Autodesk Inventor part; units mm, degrees
ref_plane "Work Plane1" through (0.508, 0.508, 2.286) normal (0, 0, 1) x (1, 0, 0)
ref_plane "Work Plane2" through (0.508, 0.508, 2.286) normal (0, 0, 1) x (1, 0, 0)
ref_plane "Work Plane3" through (0.508, 0.508, 4.826) normal (0, 0, 1) x (1, 0, 0)
sketch "Sketch1" plane through (0, 0, 0) normal (0, 0, 1) x (1, 0, 0)
  line L0 (0, 87.3125) -> (163.83, 87.3125)
  line L1 (163.83, 87.3125) -> (163.83, 0)
  line L2 (163.83, 0) -> (0, 0)
  line L3 (0, 0) -> (0, 87.3125)
  dimension "d0" = 163.83
  dimension "d1" = 87.3125
extrude "Extrusion1" add sketch "Sketch1" along normal blind 2.54
sketch "Sketch2" plane through (0, 0, 2.54) normal (0, 0, 1) x (1, 0, 0)
  point P0 (0, 0)
fillet "Fillet1" radius 20.6375 1 edges at (163.83, 87.3125, 1.27)
fillet "Fillet2" radius 20.6375 1 edges at (0, 87.3125, 1.27)
sketch "Sketch8" plane through (0, 0, 2.54) normal (0, 0, 1) x (1, 0, 0)
  point P0 (0, 0)
sketch "Sketch11" plane through (0, 0, 2.54) normal (0, 0, 1) x (1, 0, 0)
  point P0 (0, 0)
sketch "Sketch15" plane through (0, 0, 2.54) normal (0, 0, 1) x (1, 0, 0)
  line L0 (83.566, 56.2102) -> (136.1122, 56.2102)
  line L1 (136.1122, 56.2102) -> (136.1122, 16.51)
  line L2 (136.1122, 16.51) -> (83.566, 16.51)
  line L3 (83.566, 16.51) -> (83.566, 56.2102)
  line L4 (0, 0) -> (163.83, 0)
  line L5 (163.83, 0) -> (163.83, 66.675)
  dimension "d136" = 52.5463
  dimension "d137" = 16.51
  dimension "d151" = 39.7002
  dimension "d184" = 27.7177
extrude "Extrusion6" add sketch "Sketch15" along normal blind 5.08
shell "Shell5" thickness 0.762 removed faces 1 at (101.0814, 42.9768, 7.62)
sketch "Sketch16" plane through (0, 0, 2.54) normal (0, 0, 1) x (1, 0, 0)
  line L0 (103.124, 82.5754) -> (135.89, 82.5754)
  line L1 (135.89, 82.5754) -> (135.89, 56.2102)
  line L2 (135.89, 56.2102) -> (103.124, 56.2102)
  line L3 (103.124, 56.2102) -> (103.124, 82.5754)
  arc A0 (163.83, 66.675) -> (143.1925, 87.3125) centre (143.1925, 66.675) ccw
  line L4 (136.1122, 56.2102) -> (83.566, 56.2102)
  point P0 (0, 0)
  dimension "d62" = 32.766
  dimension "d63" = 26.3652
  dimension "d183" = 27.94
  dimension "d231" = 0
extrude "Extrusion7" add sketch "Sketch16" along normal blind 5.08
shell "Shell6" thickness 0.762 removed faces 1 at (124.968, 73.787, 7.62)
sketch "Sketch20" plane through (0, 0, 2.54) normal (0, 0, 1) x (1, 0, 0)
  circle A0 centre (60.325, 76.2) radius 4.445
  line L0 (0, 66.675) -> (0, 0)
  line L1 (103.124, 87.3125) -> (20.6375, 87.3125)
  point P0 (103.124, 82.5754)
  point P1 (20.6375, 87.3125)
  dimension "d77" = 8.89
  dimension "d138" = 60.325
  dimension "d150" = 11.1125
sketch "Sketch24" plane through (0, 0, 2.54) normal (0, 0, 1) x (1, 0, 0)
  line L0 (0, 0) -> (83.7565, 0)
  line L1 (83.7565, 0) -> (83.7565, 66.3575)
  line L2 (83.7565, 66.3575) -> (0, 66.3575)
  line L3 (0, 66.3575) -> (0, 0)
  line L4 (103.124, 87.3125) -> (20.6375, 87.3125)
  point P0 (103.124, 82.5754)
  point P1 (20.6375, 87.3125)
  dimension "d114" = 83.7565
  dimension "d210" = 20.955
extrude "Extrusion13" add sketch "Sketch24" along normal blind 7.62
sketch "Sketch25" plane through (0, 0, 2.54) normal (0, 0, 1) x (1, 0, 0)
  circle A0 centre (57.2977, 68.2625) radius 1.5875
  line L0 (0, 66.675) -> (0, 66.3575)
  circle A1 centre (63.6477, 68.2625) radius 1.5875
  line L1 (103.124, 87.3125) -> (20.6375, 87.3125)
  point P0 (0, 0)
  point P1 (103.124, 82.5754)
  point P2 (20.6375, 87.3125)
  dimension "d126" = 3.175
  dimension "d139" = 57.2977
  dimension "d141" = 6.35
  dimension "d149" = 19.05
sketch "Sketch27" plane through (0, 0, 2.54) normal (0, 0, 1) x (1, 0, 0)
  line L0 (62.5475, 79.375) -> (72.7075, 79.375)
  line L1 (72.7075, 79.375) -> (72.7075, 73.025)
  line L2 (72.7075, 73.025) -> (62.5475, 73.025)
  line L3 (62.5475, 73.025) -> (62.5475, 79.375)
  arc A0 (20.6375, 87.3125) -> (0, 66.675) centre (20.6375, 66.675) ccw
  point P0 (0, 0)
  dimension "d181" = 41.91
  dimension "d182" = 10.16
ref_plane "Work Plane1" through (0.508, 0.508, 2.286) normal (0, 0, 1) x (1, 0, 0)
sketch "Sketch28" plane through (0.508, 0.508, 2.286) normal (0, 0, 1) x (1, 0, 0)
  circle A0 centre (57.15, 48.7045) radius 1.5875
  circle A1 centre (56.7897, 67.7545) radius 1.5875
  circle A2 centre (63.5, 48.7045) radius 1.5875
  circle A3 centre (62.992, 67.7545) radius 1.5875
  point P0 (-0.508, -0.508)
  dimension "d154" = 19.05
  dimension "d155" = 3.175
  dimension "d156" = 19.05
  dimension "d157" = 6.35
ref_plane "Work Plane2" through (0.508, 0.508, 2.286) normal (0, 0, 1) x (1, 0, 0)
sketch "Sketch29" plane through (0.508, 0.508, 2.286) normal (0, 0, 1) x (1, 0, 0)
  line L0 (82.7405, 64.7065) -> (0, 64.7065)
  line L1 (82.7405, 0) -> (0, 0)
  line L2 (0, 64.7065) -> (82.7405, 64.7065)
  line L3 (82.7405, 64.7065) -> (82.7405, 0)
  line L4 (82.7405, 0) -> (0, 0)
  line L5 (0, 0) -> (0, 64.7065)
  point P0 (-0.508, -0.508)
  point P1 (84.836, 62.484)
extrude "Extrusion16" add sketch "Sketch29" along normal blind 2.54
ref_plane "Work Plane3" through (0.508, 0.508, 4.826) normal (0, 0, 1) x (1, 0, 0)
sketch "Sketch30" plane through (0.508, 0.508, 4.826) normal (0, 0, 1) x (1, 0, 0)
  circle A0 centre (57.15, 48.7045) radius 3.175
  circle A1 centre (63.5, 48.7045) radius 3.175
  circle A2 centre (56.7897, 67.7545) radius 1.5875
  circle A3 centre (62.992, 67.7545) radius 1.5875
  point P0 (-0.508, -0.508)
  dimension "d162" = 6.35
  dimension "d163" = 19.05
  dimension "d164" = 19.05
sketch "Sketch33" plane through (20.6375, 86.5505, 0.762) normal (0, 0, 1) x (1, 0, 0)
  line L0 (63.6905, -69.2785) -> (63.6905, -31.1023)
  line L1 (114.7127, -69.2785) -> (63.6905, -69.2785)
  line L2 (63.6905, -31.1023) -> (114.7127, -31.1023)
  line L3 (114.7127, -31.1023) -> (114.7127, -69.2785)
  line L4 (114.7127, -69.2785) -> (63.6905, -69.2785)
  line L5 (63.6905, -69.2785) -> (63.6905, -31.1023)
  point P0 (-20.6375, -86.5505)
extrude "Extrusion20" add sketch "Sketch33" along normal blind 1.778
sketch "Sketch34" plane through (0, 0, 0) normal (0, 0, -1) x (-1, 0, 0)
  line L0 (-163.83, 0) -> (0, 0)
  line L1 (0, 0) -> (0, 87.3125)
  line L2 (0, 87.3125) -> (-163.83, 87.3125)
  line L3 (-163.83, 87.3125) -> (-163.83, 0)
  point P0 (0, 0)
extrude "Extrusion21" add sketch "Sketch34" against normal blind 2.54
extrude "Extrusion22" cut sketch "Sketch20" against normal blind 7.62
extrude "Extrusion23" cut sketch "Sketch25" against normal blind 7.62
extrude "Extrusion24" cut sketch "Sketch28" along normal mid plane 7.62 contours A0 | A2
extrude "Extrusion25" cut sketch "Sketch27" against normal blind 7.62
fillet "Fillet4" radius 20.6375 1 edges at (163.83, 87.3125, 1.27)
fillet "Fillet5" radius 20.6375 1 edges at (0, 87.3125, 1.27)
sketch "Sketch35" plane through (0, 0, 2.54) normal (0, 0, 1) x (1, 0, 0)
  line L0 (135.3502, 17.272) -> (84.328, 17.272)
  line L1 (135.3502, 17.272) -> (162.2742, 17.272)
  line L2 (162.2742, 17.272) -> (162.2742, 66.802)
  line L3 (162.2742, 66.802) -> (135.3502, 66.802)
  line L4 (135.3502, 66.802) -> (135.3502, 17.272)
  point P0 (0, 0)
  point P1 (85.344, 22.352)
  dimension "d199" = 26.924
  dimension "d200" = 49.53
extrude "Extrusion26" add sketch "Sketch35" along normal blind 5.08
sketch "Sketch36" plane through (0, 0, 7.62) normal (0, 0, 1) x (1, 0, 0)
  line L0 (136.6202, 65.532) -> (160.4327, 65.532)
  line L1 (160.4327, 65.532) -> (160.4327, 14.732)
  line L2 (160.4327, 14.732) -> (136.6202, 14.732)
  line L3 (136.6202, 14.732) -> (136.6202, 65.532)
  line L4 (135.3502, 55.4482) -> (135.3502, 17.272)
  line L5 (162.2742, 66.802) -> (135.89, 66.802)
  line L6 (136.1122, 17.272) -> (162.2742, 17.272)
  point P0 (0, 0)
  point P1 (135.3502, 66.802)
  dimension "d203" = 23.8125
  dimension "d204" = 1.27
  dimension "d205" = 1.27
  dimension "d207" = 50.8
extrude "Extrusion27" cut sketch "Sketch36" against normal blind 5.08
sketch "Sketch37" plane through (0, 0, 10.16) normal (0, 0, 1) x (1, 0, 0)
  line L0 (0.762, 3.048) -> (83.5152, 3.048)
  line L1 (83.5152, 3.048) -> (83.5152, 65.3859)
  line L2 (83.5152, 65.3859) -> (0.762, 65.386)
  line L3 (0.762, 65.386) -> (0.762, 3.048)
  line L4 (0, 66.3575) -> (0, 0)
  line L5 (0, 0) -> (83.7565, 0)
  dimension "d211" = 82.7532
  dimension "d212" = 62.3379
  dimension "d213" = 0.762
  dimension "d214" = 3.048
extrude "Extrusion28" cut sketch "Sketch37" against normal blind 7.62
extrude "Extrusion29" cut sketch "Sketch30" against normal blind 2.54 contours A0 | A1
sketch "Sketch38" plane through (0, 0, 2.54) normal (0, 0, 1) x (1, 0, 0)
  line L0 (163.83, 0) -> (0, 0)
  line L1 (163.83, 0) -> (84.1375, 0)
  line L2 (84.1375, 0) -> (84.1375, 16.51)
  line L3 (84.1375, 16.51) -> (163.83, 16.51)
  line L4 (163.83, 16.51) -> (163.83, 0)
  dimension "d229" = 16.51
extrude "Extrusion30" cut sketch "Sketch38" against normal blind 12.7
sketch "Sketch39" plane through (0, 0, 7.62) normal (0, 0, 1) x (1, 0, 0)
  line L0 (83.7565, 66.3575) -> (83.7565, 56.2102)
  line L1 (83.7565, 56.2102) -> (84.328, 56.2102)
  line L2 (84.328, 56.2102) -> (84.328, 0)
  line L3 (84.328, 0) -> (83.7565, 0)
  line L4 (83.7565, 0) -> (83.7565, 56.2102)
  line L5 (84.328, 17.272) -> (84.328, 55.4482)
  line L6 (83.7565, 0) -> (84.1375, 0)
  point P0 (0, 0)
  dimension "d221" = 0
  dimension "d230" = 0
extrude "Extrusion31" add sketch "Sketch39" along normal blind 2.54 and the other way blind 7.62
sketch "Sketch40" plane through (0, 0, 10.16) normal (0, 0, 1) x (1, 0, 0)
  line L0 (84.328, 0) -> (84.328, 56.2102)
  line L1 (0, 0) -> (84.328, 0)
  line L2 (84.328, 0) -> (84.328, 2.032)
  line L3 (84.328, 2.032) -> (0, 2.032)
  line L4 (0, 2.032) -> (0, 0)
  line L5 (83.5152, 3.048) -> (0.762, 3.048)
  dimension "d226" = 1.016
extrude "Extrusion32" cut sketch "Sketch40" against normal blind 12.7
properties part number "Base Plate 2"
Geometry check sheet. Reference: the model listing, model coordinates, mm. A direction names the side the tool comes from. Round coordinates to 2 decimals unless told otherwise and drop trailing zeros. Loops run counter-clockwise (first coordinate to the right, second up) from the corner with the lowest first, then second, coordinate; pieces in that order, holes last. Notation, with made-up numbers: (70, 29.5) - (121, 29.5) arc R12 cw to (121, 36.5) - close; hole circle Ø3 at (33, 7.5). An arc over 180 degrees is marked (long way). Write item = value, one per line. Start each with the question number.
1. Section check D-D on x = 78. Enter the section's corners in (y, z), then the cut area to 3 significant figures.
2. Thickness scan on line 1 (Y direction, x = 109.5, z = 4.5); line 2 (X direction, y = 52.5, z = 7.5); line 3 (X direction, y = 65.5, z = 3.5). Record the ranges inside material, lowest first.
3. Section check A-A on z = 5.25. Give the number of separate pieces and of enclosed holes in the cut face, then the cut area to 3 significant figures.
4. Depth check by flat-ended pin: pin 1 (6 mm diameter, centred on y = 22.5, z = 8, fed in from -X); pin 2 (6 mm diameter, centred on x = 52.5, z = 7, fed in from +Y); pin 3 (2.5 mm diameter, centred on y = 52.5, z = 5, fed in from +X); pin 4 (2.5 mm diameter, centred on x = 63.65, y = 68.26, fed in from +Z). Enter the tip coordinate at first touch or a pass-through.
5. Section check B-B on y = 76.2. Enter the section's corners in (x, z), then the cut area to 3 significant figures.
6. Set-up check for faces 1 (the face through (119, 82.575, 5)), 2 (the face through (110, 17.272, 5)), 3 (the face through (161, 42, 7.62)), 4 (the face through (83.756, 61, 6)): record each of +Z, -Z, +X, -X, +Y, -Y from which the full face is reachable in a straight line by a thin tool's end or side.
7. Mould release check, pull along Y, two halves, no side actions. Record for faces 5 (the face through (136.62, 41, 5)), 6 (the face through (148, 65.532, 5)), 7 (the face through (42, 35, 2.54)): released by +Y, released by -Y, zero draft, split by the parting line, or undercut.
8. Section check C-C on y = 22.5. Enter the section's corners in (x, z).
Working result:
q1.outline = (2.03, 0) - (87.31, 0) - (87.31, 2.54) - (66.36, 2.54) - (66.36, 10.16) - (65.39, 10.16) - (65.39, 2.54) - (3.05, 2.54) - (3.05, 10.16) - (2.03, 10.16) - close
q1.area = 232 mm^2
q2.line_1 = 16.51 to 17.27, 55.45 to 56.21, 81.81 to 82.58
q2.line_2 = 0 to 0.76, 83.52 to 84.33, 135.35 to 136.62, 160.43 to 162.27
q2.line_3 = 0 to 83.76, 103.12 to 103.89, 135.13 to 136.62, 160.43 to 162.27
q3.separate_pieces = 1
q3.enclosed_holes = 3
q3.area = 581 mm^2
q4.pin_1 = 0
q4.pin_2 = 66.36
q4.pin_3 = 162.27
q4.pin_4 = through
q5.outline = (2.33, 0) - (55.88, 0) - (55.88, 2.54) - (2.33, 2.54) - close; (72.71, 0) - (161.5, 0) - (161.5, 2.54) - (135.89, 2.54) - (135.89, 7.62) - (135.13, 7.62) - (135.13, 2.54) - (103.89, 2.54) - (103.89, 7.62) - (103.12, 7.62) - (103.12, 2.54) - (72.71, 2.54) - close
q5.area = 369 mm^2
q6.face_1 = +Z, +X, -X, +Y
q6.face_2 = +Z
q6.face_3 = +Z, +X, +Y, -Y
q6.face_4 = +Z, +Y
q7.face_5 = zero draft
q7.face_6 = released by -Y
q7.face_7 = undercut
q8.outline = (0, 0) - (163.83, 0) - (163.83, 2.54) - (162.27, 2.54) - (162.27, 7.62) - (160.43, 7.62) - (160.43, 2.54) - (136.62, 2.54) - (136.62, 7.62) - (135.35, 7.62) - (135.35, 2.54) - (84.33, 2.54) - (84.33, 10.16) - (83.52, 10.16) - (83.52, 2.54) - (0.76, 2.54) - (0.76, 10.16) - (0, 10.16) - close
